Part model, mm, in its own coordinate system. A direction names the side the tool comes from. Round coordinates to 2 decimals unless told otherwise and drop trailing zeros. Loops run counter-clockwise (first coordinate to the right, second up) from the corner with the lowest first, then second, coordinate; pieces in that order, holes last.
from build123d import *

# Parameters (mm, degrees)
EXTRUDE_462_REACH = 49.007
CHAMFER_1_SIZE    = 0.920175


with BuildPart() as part:
    # 草圖1 → Revolve 332 (revolve)
    with BuildSketch(Plane.XY, mode=Mode.PRIVATE) as revolve_332_sk:
        Polygon((45, 0), (45, 5), (13, 5), (12.079825, 5), (6.2, 5), (1.59, 9.61), (0, 9.61), (0, 3.464101615), (4.18, 3.464101615), (6.18, 0), align=None)
    revolve(revolve_332_sk.sketch.rotate(Axis((6.18, 0, 0), (1, 0, 0)), 180), axis=Axis((6.18, 0, 0), (1, 0, 0)))

    # 草圖2 → Extrude 462 (add, up to next)
    with BuildSketch(Plane.ZY, mode=Mode.PRIVATE) as extrude_462_sk1:
        with BuildLine():
            ThreePointArc((0, 3.464101615), (-2.449489743, -2.449489743), (3.464101615, 0))
            ThreePointArc((3.464101615, 0), (2.449489743, 2.449489743), (0, 3.464101615))
        make_face()
    extrude_462_tool1 = extrude(extrude_462_sk1.sketch, amount=-EXTRUDE_462_REACH, mode=Mode.PRIVATE) - part.part
    add(extrude_462_tool1.solids().sort_by_distance((0, 0, 0))[0])

    # 倒角1
    chamfer_1_edges = [part.edges().sort_by_distance(p)[0] for p in [
        (45, 5, 0),
    ]]
    chamfer(chamfer_1_edges, length=CHAMFER_1_SIZE)


solid = part.part
1) Wall check: line 1 along Y through (x, z) = (35, 0.75); line 2 along X through (y, z) = (7.5, -4.5); line 3 along Y through (x, z) = (36.5, -1.75). Give the ranges that are in metal, low to high.
Values:
line 1: y = -4.94 to 4.94
line 2: x = 0 to 2.45
line 3: y = -4.68 to 4.68
2) Slice it at A-A, the plane z = 0. Give the cut face in (x, y).
Values:
outline: (0, -9.61) - (1.59, -9.61) - (6.2, -5) - (44.08, -5) - (45, -4.08) - (45, 4.08) - (44.08, 5) - (6.2, 5) - (1.59, 9.61) - (0, 9.61) - close
3) Slice it at C-C, the plane x = 18. Give the cut face in (y, z), then the cut area to 3 significant figures.
Values:
outline: circle Ø10 at (0, 0)
area: 78.5 mm2
4) Tool access for faces 1 (the face through (0, 0, 0)), 2 (the face through (25, 5, 0)): list every direction of +Z, -Z, +X, -X, +Y, -Y with a clear straight run to the whole face (end or side of a thin tool).
Values:
face 1: +Z, -Z, -X, +Y, -Y
face 2: +X
5) Drop flat-ended pins along their axis: pin 1 Ø2 at (y, z) = (6, 6) entering from +X; pin 2 Ø1.5 at (x, y) = (22, 2.5) entering from +Z; pin 3 Ø2 at (x, y) = (8, -0.5) entering from -Z. Give the stop position or say it passes through.
Values:
pin 1: stops at x = 3.71
pin 2: stops at z = 4.68
pin 3: stops at z = -5
